from build123d import *

# Parameters (mm, degrees)
SKETCH1_R           = 1.6
BOSS_EXTRUDE1_DEPTH = 4


with BuildPart() as part:
    # Sketch1 → Boss-Extrude1 (new body)
    with BuildSketch(Plane.XY):
        with BuildLine():
            Line((-2.195689363, -4.492098421), (-74.069264096, 30.638931382))
            ThreePointArc((-74.069264096, 30.638931382), (-76.365673155, 37.326719165), (-69.677885371, 39.623128223))
            Line((-69.677885371, 39.623128223), (2.195689363, 4.492098421))
            ThreePointArc((2.195689363, 4.492098421), (4.492098421, -2.195689363), (-2.195689363, -4.492098421))
        make_face()
        with Locations((-71.873574734, 35.131029803)):
            Circle(SKETCH1_R, mode=Mode.SUBTRACT)
        Circle(SKETCH1_R, mode=Mode.SUBTRACT)
        with Locations((-35.936787367, 17.565514901)):
            Circle(SKETCH1_R, mode=Mode.SUBTRACT)
    extrude(amount=BOSS_EXTRUDE1_DEPTH)


solid = part.part
Model file for the job. Use its own axes, mm. Coordinates: 2 decimals unless noted, no trailing zeros. Write each loop counter-clockwise with the first axis right and the second up, starting at its lowest first coordinate (ties: lowest second). Pieces come first, ordered by that corner, then holes. Notation, with made-up numbers: (58, 79.25) -> (109, 79.25) arc R4 cw to (109, 86.25) -> close; hole circle Ø10 at (31.5, 27). An arc over 180 degrees is marked (long way). One line per item, written item: value. Start each with the question number.
1) Pull direction X, two halves, no side cores. Call faces 1 (the face through (-34.24, 22.3, 1.97)), 2 (the face through (4.539, -2.096, 1.972)), 3 (the face through (-37.63, 12.83, 1.97)), 4 (the face through (-34.46, 16.95, 1.97)): +X half, -X half, draft (parallel to the pull), parting line (faces both ways), or undercut.
2) Slice it at C-C on y = 0. Write the cut outline in (x, z), then the cut area to 3 significant figures.
3) Slice it at A-A on z = 2.65. Write the cut outline in (x, y).
4) Slice it at B-B on x = 0. Write the cut outline in (y, z).
5) Flat gauge pins, fed straight in: pin 1 Ø1 at (x, z) = (-7.5, 1) entering from -Y; pin 2 Ø2 at (x, z) = (-10, 1.5) entering from +Y; pin 3 Ø1 at (x, z) = (-37, 2) entering from -Y; pin 4 Ø4 at (x, y) = (-71.87, 35.13) entering from -Z. Where does each tip first touch, or does it go through?
6) Slice it at D-D on x = -58.5. Write the cut outline in (y, z).
7) Probe probe 1 along X at (y, z) = (36.5, 0.8); probe 2 along Y at (x, z) = (0, 0.95); probe 3 along Y at (x, z) = (-23, 3). List the from-to ranges inside material, lowest first.
Answers follow:
1. face 1: +X half
1. face 2: parting line
1. face 3: -X half
1. face 4: undercut
2. outline: (-11.39, 0) -> (-1.6, 0) -> (-1.6, 4) -> (-11.39, 4) -> close; (1.6, 0) -> (5, 0) -> (5, 4) -> (1.6, 4) -> close
2. area: 52.7 mm2
3. outline: (-74.07, 30.64) -> (-2.2, -4.49) arc R5 ccw to (2.2, 4.49) -> (-69.68, 39.62) arc R5 ccw to start; hole circle Ø3.2 at (-71.87, 35.13); hole circle Ø3.2 at (-35.94, 17.57); hole circle Ø3.2 at (0, 0)
4. outline: (-5, 0) -> (-1.6, 0) -> (-1.6, 4) -> (-5, 4) -> close; (1.6, 0) -> (5.57, 0) -> (5.57, 4) -> (1.6, 4) -> close
5. pin 1: y = -2.14
5. pin 2: y = 10.94
5. pin 3: y = 12.28
5. pin 4: z = 0
6. outline: (23.03, 0) -> (34.16, 0) -> (34.16, 4) -> (23.03, 4) -> close
7. probe 1: -76.68 to -72.7, -71.05 to -63.29
7. probe 2: -5 to -1.6, 1.6 to 5.57
7. probe 3: 5.68 to 16.81
